from build123d import *

# Parameters (mm, degrees)
SKETCH_1_W      = 10.284966626
SKETCH_1_H      = 9.380426844
EXTRUDE_1_DEPTH = 5
SKETCH_2_R      = 1.5
EXTRUDE_2_DEPTH = 5


with BuildPart() as part:
    # 草图1 → 凸台-拉伸1 (new body)
    with BuildSketch(Plane.XY):
        Rectangle(SKETCH_1_W, SKETCH_1_H)
    extrude(amount=EXTRUDE_1_DEPTH)

    # 草图2 → 凸台-拉伸2 (add)
    with BuildSketch(Plane.XZ.offset(4.690213422)):
        with Locations(Location((2.553176364, 2.478071855, 0), (0, 0, 90))):
            Circle(SKETCH_2_R)
        with Locations(Location((-2.553176364, 2.478071855, 0), (0, 0, 90))):
            Circle(SKETCH_2_R)
    extrude(amount=EXTRUDE_2_DEPTH)


solid = part.part
The listing builds one solid part. Answer for the finished solid, in the listing's coordinates (mm). A direction names the side the tool comes from. Round coordinates to 2 decimals unless told otherwise and drop trailing zeros. Order: outer loops, then holes, each group sorted by start corner. A loop starts at its lowest first (then second) coordinate and runs counter-clockwise, first axis right, second up. Notation, with made-up numbers: M 29,57.25 L 55,57.25 A14 ccw 55,75.25 Z; hole C -27.5,56 d7. An arc over 180 degrees is marked long. Answer in a Markdown table with one row per item. Add a question column.
1) Which of the six approach directions +Z, -Z, +X, -X, +Y, -Y give full straight-line access (tool end or side, diameter ignored) to faces 4 (the face through (-3, -9.69, 2)), 5 (the face through (0, -4.69, 2))?
2) The part is cut by section B-B on x = 1.25. Determine the outline of the cut face in (y, z).
3) Determine the mould class of faces 1 (the face through (3, -9.69, 2)), 2 (the face through (5.142, 0, 2)), 3 (the face through (-1.979, -7.155, 3.864)) for opening direction X: pulls with the +X half, pulls with the -X half, needs draft (parallel to the pull), parting line crosses it, or undercut.
4) Consider line 1 along Y through (x, z) = (1.5, 0.3); line 2 along Z through (x, y) = (1.25, -5). Determine where each line is inside the solid, lowest interval first. Write a range as from..to.
5) The part is cut by section C-C on y = -5.5. Determine the outline of the cut face in (x, z), plus the area to 3 significant figures.
6) The part is cut by section A-A on z = 2.85. Determine the outline of the cut face in (x, y), plus the area to 3 significant figures.
7) The part is cut by section D-D on z = 0.3. Determine the outline of the cut face in (x, y), plus the area to 3 significant figures.
Findings below:
| question | item | result |
|---|---|---|
| 1 | face 4 | +Z, -Z, +X, -X, -Y |
| 1 | face 5 | -Y |
| 2 | outline | M -9.69,1.74 L -4.69,1.74 L -4.69,0 L 4.69,0 L 4.69,5 L -4.69,5 L -4.69,3.22 L -9.69,3.22 Z |
| 3 | face 1 | needs draft |
| 3 | face 2 | pulls with the +X half |
| 3 | face 3 | undercut |
| 4 | line 1 | y = -4.69..4.69 |
| 4 | line 2 | z = 1.74..3.22 |
| 5 | outline | C -2.55,2.48 d3; C 2.55,2.48 d3 |
| 5 | area | 14.1 mm² |
| 6 | outline | M -5.14,-4.69 L -4.01,-4.69 L -4.01,-9.69 L -1.1,-9.69 L -1.1,-4.69 L 1.1,-4.69 L 1.1,-9.69 L 4.01,-9.69 L 4.01,-4.69 L 5.14,-4.69 L 5.14,4.69 L -5.14,4.69 Z |
| 6 | area | 126 mm² |
| 7 | outline | M -5.14,-4.69 L 5.14,-4.69 L 5.14,4.69 L -5.14,4.69 Z |
| 7 | area | 96.5 mm² |
